```python
from build123d import *

# Parameters (mm, degrees)
F1_DEPTH  = 457.2
F2_W      = 91.44
F2_H      = 38.1
F3_DEPTH  = 6.35
F4_W      = 45.72
F4_H      = 19.05
F5_DEPTH  = 19.05
F6_W      = 9.144
F6_H      = 19.05
F7_DEPTH  = 25.4
F9_DEPTH  = 27.94
F10_R     = 6.35
F11_DEPTH = 50.8


with BuildPart() as f1:
    # F0 (on Right) → F1 (new body)
    with BuildSketch(Plane.YZ):
        with BuildLine():
            add(Edge.make_bspline(
                [(0, 0), (7.9206921486, 0.4964849945), (41.788781698, 2.6194053072), (328.8937583875, -268.1300359687), (324.4514783657, -311.8504178384), (323.2892203585, -323.2892203585)],
                knots=[0, 0, 0, 0, 0.1839351844, 0.786488501, 1, 1, 1, 1], degree=3))
            Line((0, 0), (323.2892203585, -323.2892203585))
        make_face()
    extrude(amount=F1_DEPTH)

    # F2 (on face) → F3 (join)
    with BuildSketch(Plane(origin=(0, 0, 0), x_dir=(1, 0, 0), z_dir=(0, -0.7071067812, -0.7071067812))):
        with Locations((228.6, -228.6)):
            Rectangle(F2_W, F2_H)
    extrude(amount=F3_DEPTH)

    # F4 (on face) → F5 (join)
    with BuildSketch(Plane(origin=(0, -4.4901280605, -4.4901280605), x_dir=(1, 0, 0), z_dir=(0, -0.7071067812, -0.7071067812))):
        with Locations((228.6, -228.6)):
            Rectangle(F4_W, F4_H)
    extrude(amount=F5_DEPTH)

    # F6 (on face) → F7 (cut)
    with BuildSketch(Plane(origin=(0, -17.9605122421, -17.9605122421), x_dir=(1, 0, 0), z_dir=(0, -0.7071067812, -0.7071067812))):
        with Locations((210.312, -228.6)):
            Rectangle(F6_W, F6_H)
        with Locations((228.6, -228.6)):
            Rectangle(F6_W, F6_H)
        with Locations((246.888, -228.6)):
            Rectangle(F6_W, F6_H)
    extrude(amount=-F7_DEPTH, mode=Mode.SUBTRACT)

    # F8 (on face) → F9 (cut)
    with BuildSketch(Plane.YZ.offset(242.316)):
        with BuildLine():
            ThreePointArc((144.492320988, -165.3265151889), (148.8943740988, -162.8268771513), (153.9554431224, -162.9356992435))
            Line((153.9554431224, -162.9356992435), (150.4192900279, -159.399546149))
            Line((150.4192900279, -159.399546149), (144.492320988, -165.3265151889))
        make_face()
        with BuildLine():
            ThreePointArc((160.353521115, -169.3337772361), (160.6522372537, -170.683230139), (160.7525130788, -172.0617072797))
            ThreePointArc((160.7525130788, -172.0617072797), (160.027465626, -175.706766973), (157.9627051696, -178.7968993705))
            Line((157.9627051696, -178.7968993705), (163.8896742095, -172.8699303306))
            Line((163.8896742095, -172.8699303306), (160.353521115, -169.3337772361))
        make_face()
        with BuildLine():
            Line((150.4192900279, -186.3403145122), (157.9627051696, -178.7968993705))
            ThreePointArc((157.9627051696, -178.7968993705), (144.492320988, -178.7968993705), (144.492320988, -165.3265151889))
            Line((144.492320988, -165.3265151889), (136.9489058463, -172.8699303306))
            Line((136.9489058463, -172.8699303306), (150.4192900279, -186.3403145122))
        make_face()
    extrude(amount=-F9_DEPTH, mode=Mode.SUBTRACT)

    # F10 (on face) → F11 (cut)
    with BuildSketch(Plane(origin=(214.884, 0, 0), x_dir=(0, -1, 0), z_dir=(-1, 0, 0))):
        with Locations((-151.2275130788, -172.0617072797)):
            Circle(F10_R)
    extrude(amount=-F11_DEPTH, mode=Mode.SUBTRACT)


solid = f1.part
```
The model under review builds one solid part; all positions refer to its coordinate system, in mm. A direction names the side the tool comes from. Round coordinates to 2 decimals unless told otherwise and drop trailing zeros. Answer as a JSON object with one key per item and string values. Group by question number.
1) Mouldability with a two-part tool opening along Y and no side actions: class faces 1 (the face through (219.392, 156.267, -175.926)), 2 (the face through (274.32, 160, -164)) as released by +Y, released by -Y, zero draft, split by the parting line, or undercut.
2) For pin 1 Ø21.5 at (y, z) = (153, -166.5) entering from +X; pin 2 Ø10 at (y, z) = (134, -79) entering from -X; pin 3 Ø12 at (x, z) = (83.5, -161) entering from -Y; pin 4 Ø12 at (x, y) = (139, 89.5) entering from +Z, all flat-tipped, find the tip position at first contact; note any pin that passes through.
3) For faces 3 (the face through (237.68, 156.267, -175.926)), 4 (the face through (182.88, 160, -164)), 5 (the face through (210, 162, -162)), list the 3-axis set-ups (+Z, -Z, +X, -X, +Y, -Y) from which the entire face can be reached by the end or side of a thin tool; tool diameter is ignored.
4) For line 1 (Z direction, x = 170, y = 274); line 2 (Z direction, x = 388.5, y = 168); line 3 (Y direction, x = 340.5, z = -47.5), list the stretches that pass through material, from the lowest coordinate up. Write a range as [from, to].
Result set:
{
 "1": {"face 1": "undercut", "face 2": "zero draft"},
 "2": {"pin 1": "x = 457.2", "pin 2": "through", "pin 3": "y = 155", "pin 4": "z = -46.98"},
 "3": {"face 3": "+X, -X", "face 4": "-Z, -X, -Y", "face 5": "none"},
 "4": {"line 1": "[-274, -230.46]", "line 2": "[-168, -122.09]", "line 3": "[47.5, 84.13]"}
}
